Can you work these out from the model? Positions are in its coordinate system, mm. Face numbers are marked on the shaded views. A direction names the side the tool comes from. Round coordinates to 2 decimals unless told otherwise and drop trailing zeros. Loops run counter-clockwise (first coordinate to the right, second up) from the corner with the lowest first, then second, coordinate; pieces in that order, holes last.
(1) I want a section at D-D on x = 0. Write out the boundary of the cut face in (y, z).
(2) I want a section at B-B on y = 25. Write out the boundary of the cut face in (x, z), plus the area to 3 significant figures.
(3) Thinking about a two-plate mould opening in X: for the marked faces 3 and 4, which applies, released by +X, released by -X, zero draft, split by the parting line, or undercut?
(4) Will these pins go through, and if not, where does the flat tip stop? pin 1 Ø4 at (x, y) = (-15.5, 9.5) entering from -Z; pin 2 Ø17.5 at (x, z) = (-2, 3) entering from +Y.
(5) I want a section at A-A on x = 15.5. Write out the boundary of the cut face in (y, z).
(6) Which directions (+Z, -Z, +X, -X, +Y, -Y) give clear straight access to the entire face, cutting with the end or side of a thin tool? Please do the marked faces 1 and 2.
(7) I want a section at C-C on z = -10. Write out the boundary of the cut face in (x, y).
(8) If I drill on line 1 along Y through (x, z) = (15.5, 16.85); line 2 along X through (y, z) = (1, -10); line 3 along Z through (x, y) = (14, 44), over which ranges is the centre line in solid material (lowest first)?
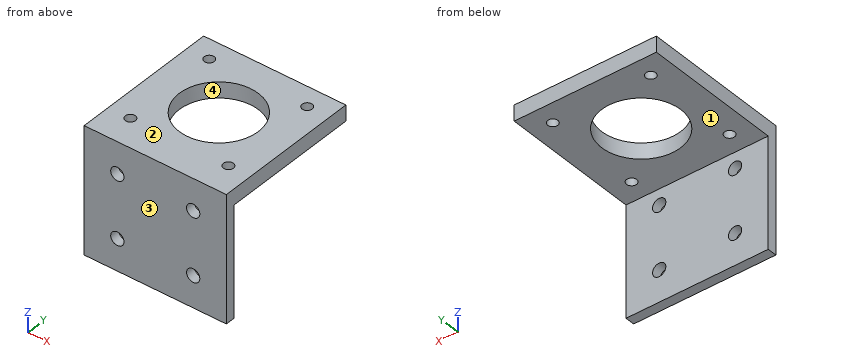
from build123d import *

# Parameters (mm, degrees)
SKETCH_2_W          = 45
SKETCH_2_H          = 40
EXTRUDE_1_DEPTH     = 3
SKETCH_3_R          = 2.1
CUT_EXTRUDE_1_DEPTH = 31.253099015
SKETCH_4_W          = 45
SKETCH_4_H          = 5
EXTRUDE_2_DEPTH     = 44
SKETCH_6_R          = 1.6
SKETCH_6_R_2        = 12.5
CUT_EXTRUDE_3_DEPTH = 63.77141069


with BuildPart() as part:
    # ｽｹｯﾁ2 → ﾎﾞｽ - 押し出し1 (new body)
    with BuildSketch(Plane(origin=(0, 0, 0), x_dir=(1, 0, 0), z_dir=(0, 1, 0))):
        Rectangle(SKETCH_2_W, SKETCH_2_H)
    extrude(amount=EXTRUDE_1_DEPTH)

    # ｽｹｯﾁ3 → ｶｯﾄ - 押し出し1 (cut, through all)
    with BuildSketch(Plane(origin=(0, 3, 0), x_dir=(1, 0, 0), z_dir=(0, 1, 0))):
        with Locations(Location((-12, 10, 0), (0, 0, 270))):
            Circle(SKETCH_3_R)
        with Locations(Location((12, 10, 0), (0, 0, 90))):
            Circle(SKETCH_3_R)
        with Locations(Location((12, -10, 0), (0, 0, 270))):
            Circle(SKETCH_3_R)
        with Locations(Location((-12, -10, 0), (0, 0, 90))):
            Circle(SKETCH_3_R)
    extrude(amount=-CUT_EXTRUDE_1_DEPTH, mode=Mode.SUBTRACT)

    # ｽｹｯﾁ4 → ﾎﾞｽ - 押し出し2 (add)
    with BuildSketch(Plane(origin=(0, 3, 0), x_dir=(1, 0, 0), z_dir=(0, 1, 0))):
        with Locations((0, -17.5)):
            Rectangle(SKETCH_4_W, SKETCH_4_H)
    extrude(amount=EXTRUDE_2_DEPTH)

    # ｽｹｯﾁ6 → ｶｯﾄ - 押し出し3 (cut, through all)
    with BuildSketch(Plane(origin=(0, 0, 15), x_dir=(-1, 0, 0), z_dir=(0, 0, -1))):
        with Locations((-15.5, 40.5)):
            Circle(SKETCH_6_R)
        with Locations(Location((15.5, 40.5, 0), (0, 0, 180))):
            Circle(SKETCH_6_R)
        with Locations((15.5, 9.5)):
            Circle(SKETCH_6_R)
        with Locations(Location((-15.5, 9.5, 0), (0, 0, 180))):
            Circle(SKETCH_6_R)
        with Locations((0, 25)):
            Circle(SKETCH_6_R_2)
    extrude(amount=-CUT_EXTRUDE_3_DEPTH, mode=Mode.SUBTRACT)


solid = part.part
Filled sheet:
1. outline: (0, -20) - (3, -20) - (3, 15) - (12.5, 15) - (12.5, 20) - (0, 20) - close; (37.5, 15) - (47, 15) - (47, 20) - (37.5, 20) - close
2. outline: (-22.5, 15) - (-12.5, 15) - (-12.5, 20) - (-22.5, 20) - close; (12.5, 15) - (22.5, 15) - (22.5, 20) - (12.5, 20) - close
2. area: 100 mm2
3. face 3: zero draft
3. face 4: undercut
4. pin 1: stops at z = 15
4. pin 2: stops at y = 3
5. outline: (0, -20) - (3, -20) - (3, 15) - (7.9, 15) - (7.9, 20) - (0, 20) - close; (11.1, 15) - (38.9, 15) - (38.9, 20) - (11.1, 20) - close; (42.1, 15) - (47, 15) - (47, 20) - (42.1, 20) - close
6. face 1: -Z, +X, -X, +Y
6. face 2: +Z, +X, -X, +Y, -Y
7. outline: (-22.5, 0) - (-14.1, 0) - (-14.1, 3) - (-22.5, 3) - close; (-9.9, 0) - (9.9, 0) - (9.9, 3) - (-9.9, 3) - close; (14.1, 0) - (22.5, 0) - (22.5, 3) - (14.1, 3) - close
8. line 1: y = 0 to 7.9, 11.1 to 38.9, 42.1 to 47
8. line 2: x = -22.5 to -14.1, -9.9 to 9.9, 14.1 to 22.5
8. line 3: z = 15 to 20
